```python
from build123d import *

# Parameters (mm, degrees)
SKETCH1_R                = 34.458333333
SKETCH1_R_2              = 3
BOSS_EXTRUDE1_DEPTH      = 5.8
SKETCH2_R                = 0.79375
CUT_EXTRUDE1_DEPTH       = 50.075385604
M3_CLEARANCE_HOLE1_D     = 3.2
M3_CLEARANCE_HOLE1_DEPTH = 12.7
M3_CLEARANCE_HOLE1_TIP   = 0.96137699


with BuildPart() as part:
    # Sketch1 → Boss-Extrude1 (new body)
    with BuildSketch(Plane.XY):
        Circle(SKETCH1_R)
        Circle(SKETCH1_R_2, mode=Mode.SUBTRACT)
    extrude(amount=BOSS_EXTRUDE1_DEPTH)

    # Sketch2 → Cut-Extrude1 (cut, through all)
    with BuildSketch(Plane.XY.offset(5.8)):
        with Locations((0, 12)):
            Circle(SKETCH2_R)
        with Locations((12, 0)):
            Circle(SKETCH2_R)
        with Locations((0, -12)):
            Circle(SKETCH2_R)
        with Locations((-12, 0)):
            Circle(SKETCH2_R)
        with Locations((-18, 26)):
            Circle(SKETCH2_R)
        with Locations((26, 18)):
            Circle(SKETCH2_R)
        with Locations((18, -26)):
            Circle(SKETCH2_R)
        with Locations((-26, -18)):
            Circle(SKETCH2_R)
    extrude(amount=-CUT_EXTRUDE1_DEPTH, mode=Mode.SUBTRACT)

    # M3 Clearance Hole1
    with Locations(Plane.XY.offset(5.8)):
        with Locations((-6, 0), (6, 0)):
            Hole(M3_CLEARANCE_HOLE1_D / 2, depth=M3_CLEARANCE_HOLE1_DEPTH)
            with Locations((0, 0, -(M3_CLEARANCE_HOLE1_DEPTH + M3_CLEARANCE_HOLE1_TIP / 2))):  # 118° drill point
                Cone(0, M3_CLEARANCE_HOLE1_D / 2, M3_CLEARANCE_HOLE1_TIP, mode=Mode.SUBTRACT)


solid = part.part
```
Check sheet for the modelled part. Datum: model origin and axes. Units: mm. Coordinates: 2 decimals unless noted, no trailing zeros. Loops run counter-clockwise (first coordinate to the right, second up) from the corner with the lowest first, then second, coordinate; pieces in that order, holes last.
1) Material ranges on probe 1 along Y at (x, z) = (0, 4.5); probe 2 along X at (y, z) = (1, 1.6); probe 3 along Y at (x, z) = (-26, 2.65), recorded low to high.
2) Sectioned sample at B-B (x = 18). Record the boundary of the cut face in (y, z).
3) Release check for a two-part mould opening along Y. For faces 1 (the face through (32.867, 10.35, 2.859)), 2 (the face through (0, -7, 0)), 3 (the face through (12.757, 0.238, 2.941)) record: released by +Y, released by -Y, zero draft, split by the parting line, or undercut.
4) Sectioned sample at A-A (z = 3.25). Count the separate pieces of the cut face and the enclosed holes in it, and give its area (3 significant figures).
5) Gauge pin test, flat ends, axial feed: pin 1 (1 mm diameter, centred on x = 27, z = 2.5, fed in from +Y); pin 2 (2 mm diameter, centred on y = -17.5, z = 1.5, fed in from -X); pin 3 (1.3 mm diameter, centred on x = -12, y = 0, fed in from +Z); pin 4 (1.5 mm diameter, centred on y = -3.5, z = 2, fed in from -X). Record the tip position at first contact, or that the pin passes through.
6) Sectioned sample at D-D (x = 0). Record the boundary of the cut face in (y, z).
Check sheet entries:
1. probe 1: y = -34.46 to -12.79, -11.21 to -3, 3 to 11.21, 12.79 to 34.46
1. probe 2: x = -34.44 to -7.25, -4.75 to -2.83, 2.83 to 4.75, 7.25 to 34.44
1. probe 3: y = -22.61 to -18.79, -17.21 to 22.61
2. outline: (-29.38, 0) - (-26.79, 0) - (-26.79, 5.8) - (-29.38, 5.8) - close; (-25.21, 0) - (29.38, 0) - (29.38, 5.8) - (-25.21, 5.8) - close
3. face 1: split by the parting line
3. face 2: zero draft
3. face 3: undercut
4. separate pieces: 1
4. enclosed holes: 11
4. area: 3,670 mm2
5. pin 1: stops at y = 22.03
5. pin 2: stops at x = -30.25
5. pin 3: passes through
5. pin 4: stops at x = -34.35
6. outline: (-34.46, 0) - (-12.79, 0) - (-12.79, 5.8) - (-34.46, 5.8) - close; (-11.21, 0) - (-3, 0) - (-3, 5.8) - (-11.21, 5.8) - close; (3, 0) - (11.21, 0) - (11.21, 5.8) - (3, 5.8) - close; (12.79, 0) - (34.46, 0) - (34.46, 5.8) - (12.79, 5.8) - close
